Geometry: final body of the model. Coordinates: model frame, mm. Face numbers are marked on the shaded views. A direction names the side the tool comes from. Coordinates: 2 decimals unless noted, no trailing zeros. Write each loop counter-clockwise with the first axis right and the second up, starting at its lowest first coordinate (ties: lowest second). Pieces come first, ordered by that corner, then holes. Notation, with made-up numbers: (89, 39) -> (129, 39) arc R16 cw to (129, 50) -> close; hole circle Ø10 at (13, 27.5). An arc over 180 degrees is marked (long way). One line per item, written item: value.
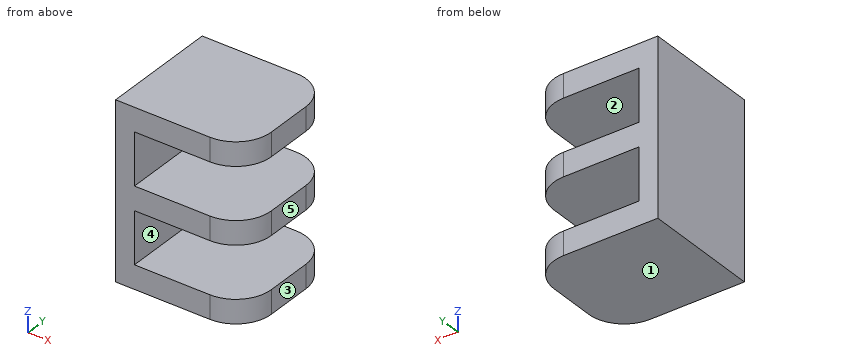
Solid Edge part; units mm, degrees
sketch "Sketch1" plane through (0, 0, 0) normal (0, -1, 0) x (1, 0, 0)
  line L0 (36.3551, 37) -> (36.3551, 27)
  line L1 (36.3551, 27) -> (-10.6407, 27)
  line L2 (-10.6407, 27) -> (-10.6407, 5)
  line L3 (-10.6407, 5) -> (36.3551, 5)
  line L4 (36.3551, 5) -> (36.3551, -5)
  line L5 (36.3551, -5) -> (-10.6407, -5)
  line L6 (-10.6407, -5) -> (-10.6407, -27)
  line L7 (-10.6407, -27) -> (36.3551, -27)
  line L8 (36.3551, -27) -> (36.3551, -37)
  line L9 (36.3551, -37) -> (-18.6407, -37)
  line L10 (-18.6407, -37) -> (-18.6407, 37)
  line L11 (-18.6407, 37) -> (36.3551, 37)
  dimension "D1" = 10.6407
  dimension "D2" = 36.3551
extrude "Protrusion1" add sketch "Sketch1" along normal mid plane 50
fillet "Round_2" radius 15 6 edges at (36.3551, -25, 32) (36.3551, -25, 0) (36.3551, -25, -32) (36.3551, 25, -32) (36.3551, 25, 0) (36.3551, 25, 32)
(1) Section D-D (x = 33). Return the cut outline in (y, z), then the cut area to 3 significant figures.
Responses:
outline: (-19.45, -37) -> (19.45, -37) -> (19.45, -27) -> (-19.45, -27) -> close; (-19.45, -5) -> (19.45, -5) -> (19.45, 5) -> (-19.45, 5) -> close; (-19.45, 27) -> (19.45, 27) -> (19.45, 37) -> (-19.45, 37) -> close
area: 1,170 mm2
(2) First-contact query: pin 1 (11 mm diameter, centred on y = 10.5, z = 19, fed in from +X). Flat tip, straight axial feed; report the tip coordinate or a pass-through.
Responses:
pin 1: stops at x = -10.64
(3) Pull-direction query (Z, two-part tool) for the marked faces 1, 2 and 3; classes: released by +Z, released by -Z, zero draft, split by the parting line, or undercut.
Responses:
face 1: released by -Z
face 2: undercut
face 3: zero draft
(4) Reachability of the marked faces 4 and 5 from +Z, -Z, +X, -X, +Y, -Y: full face, straight path, thin tool, end or side. Return the list, or none.
Responses:
face 4: +X, +Y, -Y
face 5: +Z, -Z, +X, +Y, -Y
(5) Line query: line 1 (Z direction, x = 18, y = -6); line 2 (X direction, y = -4, z = -7.5); line 3 (Y direction, x = 29, z = -29). Output: solid intervals per line, ascending. Write a range as [from, to].
Responses:
line 1: z = [-37, -27], [-5, 5], [27, 37]
line 2: x = [-18.64, -10.64]
line 3: y = [-22.91, 22.91]
(6) Section A-A (x = 10.5). Return the cut outline in (y, z), then the cut area to 3 significant figures.
Responses:
outline: (-25, -37) -> (25, -37) -> (25, -27) -> (-25, -27) -> close; (-25, -5) -> (25, -5) -> (25, 5) -> (-25, 5) -> close; (-25, 27) -> (25, 27) -> (25, 37) -> (-25, 37) -> close
area: 1,500 mm2
(7) Section C-C (z = -32). Return the cut outline in (x, y).
Responses:
outline: (-18.64, -25) -> (21.36, -25) arc R15 ccw to (36.36, -10) -> (36.36, 10) arc R15 ccw to (21.36, 25) -> (-18.64, 25) -> close
(8) Section B-B (y = 6.5). Return the cut outline in (x, z).
Responses:
outline: (-18.64, -37) -> (36.36, -37) -> (36.36, -27) -> (-10.64, -27) -> (-10.64, -5) -> (36.36, -5) -> (36.36, 5) -> (-10.64, 5) -> (-10.64, 27) -> (36.36, 27) -> (36.36, 37) -> (-18.64, 37) -> close
